Check sheet for the modelled part. Datum: model origin and axes. Units: mm. A direction names the side the tool comes from. Round coordinates to 2 decimals unless told otherwise and drop trailing zeros. Order: outer loops, then holes, each group sorted by start corner. A loop starts at its lowest first (then second) coordinate and runs counter-clockwise, first axis right, second up.
Q1. Cross-section at B-B on x = 0. Record the cut outline in (y, z), then the cut area to 3 significant figures.
Q2. Cross-section at C-C on y = 0. Record the cut outline in (x, z).
Q3. Set-up check for faces 4 (the flat face through (0, 36.976, 15)), 5 (the flat face through (-2.304, 19, 15)), 6 (the flat face through (8, -16, 27.5)), 7 (the flat face through (8, 16, 2.5)), 8 (the flat face through (20, 2.034, 15)): record each of +Z, -Z, +X, -X, +Y, -Y from which the full face is reachable in a straight line by a thin tool's end or side.
Q4. Mould release check, pull along X, two halves, no side actions. Record for faces 1 (the flat face through (0, -36.976, 15)), 2 (the flat face through (2.304, -20, 15)), 3 (the cylindrical face through (3, 0, 15)): +X half, -X half, draft (parallel to the pull), parting line (faces both ways), or undercut.
Q5. Depth check by flat-ended pin: P1, Ø1, axis at y = -5.5, z = 20.5, coming from the -X side; P2, Ø1, axis at x = 29, z = 8, coming from the -Y side; P3, Ø4.5, axis at y = 0.5, z = 15.5, coming from the +X side. Enter the tip coordinate at first touch or a pass-through.
Q6. Cross-section at D-D on y = -15.5. Record the cut outline in (x, z), then the cut area to 3 significant figures.
Q7. Cross-section at A-A on z = 19.5. Record the cut outline in (x, y).
Q8. Scan lines: probe 1 along Y at (x, z) = (0, 24); probe 2 along Z at (x, y) = (-9, -11.5); probe 3 along Y at (x, z) = (-33.5, 11). Record each from-to range of solid material in increasing order.
from build123d import *

# Parameters (mm, degrees)
F0_R     = 37.5
F1_DEPTH = 2.5
F2_W     = 74.8896048808
F2_H     = 4.0678103206
F3_DEPTH = 25
F4_W     = 4.6082469635
F4_H     = 73.9512071013
F5_DEPTH = 25
F6_R     = 37.5
F7_DEPTH = 2.5
F9_D     = 6


with BuildPart() as f1:
    # F0 (on Top) → F1 (new body)
    with BuildSketch(Plane.XY):
        Circle(F0_R)
    extrude(amount=F1_DEPTH)

    # F2 (on face) → F3 (join)
    with BuildSketch(Plane.XY.offset(2.5)):
        Rectangle(F2_W, F2_H)
    extrude(amount=F3_DEPTH)

    # F4 (on face) → F5 (join)
    with BuildSketch(Plane.XY.offset(2.5)):
        Rectangle(F4_W, F4_H)
    extrude(amount=F5_DEPTH)

    # F6 (on face) → F7 (join)
    with BuildSketch(Plane.XY.offset(27.5)):
        Circle(F6_R)
    extrude(amount=F7_DEPTH)

    # F9 (through all)
    with Locations(Plane.XY.offset(30)):
        with Locations((0, 0)):
            Hole(F9_D / 2)


solid = f1.part
Results found:
1. outline: (-37.5, 0) - (-3, 0) - (-3, 30) - (-37.5, 30) - (-37.5, 27.5) - (-36.98, 27.5) - (-36.98, 2.5) - (-37.5, 2.5) - close; (3, 0) - (37.5, 0) - (37.5, 2.5) - (36.98, 2.5) - (36.98, 27.5) - (37.5, 27.5) - (37.5, 30) - (3, 30) - close
1. area: 2,040 mm2
2. outline: (-37.5, 0) - (-3, 0) - (-3, 30) - (-37.5, 30) - (-37.5, 27.5) - (-37.44, 27.5) - (-37.44, 2.5) - (-37.5, 2.5) - close; (3, 0) - (37.5, 0) - (37.5, 2.5) - (37.44, 2.5) - (37.44, 27.5) - (37.5, 27.5) - (37.5, 30) - (3, 30) - close
3. face 4: +X, -X, +Y
3. face 5: -X, +Y
3. face 6: -Y
3. face 7: +Y
3. face 8: +X, +Y
4. face 1: draft
4. face 2: +X half
4. face 3: undercut
5. P1: stops at x = -2.3
5. P2: stops at y = -2.03
5. P3: stops at x = 37.44
6. outline: (-34.15, 0) - (34.15, 0) - (34.15, 2.5) - (2.3, 2.5) - (2.3, 27.5) - (34.15, 27.5) - (34.15, 30) - (-34.15, 30) - (-34.15, 27.5) - (-2.3, 27.5) - (-2.3, 2.5) - (-34.15, 2.5) - close
6. area: 457 mm2
7. outline: (-37.44, -2.03) - (-2.3, -2.03) - (-2.3, -36.98) - (2.3, -36.98) - (2.3, -2.03) - (37.44, -2.03) - (37.44, 2.03) - (2.3, 2.03) - (2.3, 36.98) - (-2.3, 36.98) - (-2.3, 2.03) - (-37.44, 2.03) - close; hole circle Ø6 at (0, 0)
8. probe 1: y = -36.98 to -3, 3 to 36.98
8. probe 2: z = 0 to 2.5, 27.5 to 30
8. probe 3: y = -2.03 to 2.03
